Here's how the part is built. I have some questions about the finished solid (model axes, mm). A direction names the side the tool comes from. Coordinates: 2 decimals unless noted, no trailing zeros. Order: outer loops, then holes, each group sorted by start corner. A loop starts at its lowest first (then second) coordinate and runs counter-clockwise, first axis right, second up. Notation, with made-up numbers: (9, 11.5) - (40, 11.5) arc R22 ccw to (40, 40.5) - close; hole circle Ø3 at (68.5, -23.75). An arc over 180 degrees is marked (long way). Answer as CSV lines item,"result". Start each with the question number.
Item 1: I need wall thicknesses on line 1 (Z direction, x = -4, y = 2); line 2 (Z direction, x = -54, y = 4.75); line 3 (Z direction, x = -21.5, y = 6). Which ranges of each line are inside material? Lowest first, please.
Item 2: I'm going to push a flat-ended pin straight in: pin 1 (8 mm diameter, centred on x = -29.5, z = 8.5, fed in from +Y). Where does the tip first touch, or does it pass through?
Item 3: Imagine slicing it at D-D on x = -40. List the corners of the cut face in (y, z) for me, and give its area (3 significant figures).
Item 4: Imagine slicing it at C-C on y = 1. Count the separate pieces of the cut face and the enclosed holes in it, and give its area (3 significant figures).
Item 5: Imagine slicing it at A-A on x = -14. List the corners of the cut face in (y, z) for me.
Item 6: On a 3-axis mill with a long thin cutter (end or side, diameter ignored), from which of +Z, -Z, +X, -X, +Y, -Y can I reach the whole of each face in a straight line? I mean faces 1 (the face through (-31, 0, 32)), 2 (the face through (-5, 4, 19)). Say none if no direction works.
Item 7: Imagine slicing it at B-B on z = 4. List the corners of the cut face in (x, y) for me.
Item 8: We'd pull the mould along X, two halves only. Please class faces 3 (the face through (0, 4, 19)), 4 (the face through (-12.8, 4.2, 34.9)), 5 (the face through (-31, 4, 0)): pulls with the +X half, pulls with the -X half, needs draft (parallel to the pull), parting line crosses it, or undercut.
Autodesk Inventor part; units mm, degrees
ref_plane "YZ Plane" through (0, 0, 0) normal (1, 0, 0) x (0, 1, 0)
ref_plane "XZ Plane" through (0, 0, 0) normal (0, 1, 0) x (-1, 0, 0)
ref_plane "XY Plane" through (0, 0, 0) normal (0, 0, 1) x (1, 0, 0)
sketch "スケッチ1" plane through (0, 0, 0) normal (0, 1, 0) x (-1, 0, 0)
  circle A0 centre (4, 34) radius 1.5
  circle A1 centre (44, 34) radius 1.5
  circle A2 centre (24, 34) radius 1.5
  circle A3 centre (44, 4) radius 1.5
  circle A4 centre (24, 4) radius 1.5
  circle A5 centre (4, 4) radius 1.5
  circle A6 centre (14, 4) radius 1.5
  circle A7 centre (34, 4) radius 1.5
  circle A8 centre (54, 4) radius 1.5
  circle A9 centre (34, 34) radius 1.5
  circle A10 centre (54, 34) radius 1.5
  circle A11 centre (14, 34) radius 1.5
  line L0 (0, 0) -> (62, 0)
  line L1 (62, 0) -> (62, 38)
  line L2 (62, 38) -> (0, 38)
  line L3 (0, 38) -> (0, 0)
extrude "押し出し1" add sketch "スケッチ1" along normal blind 8.5
sketch "スケッチ2" plane through (0, 0, 0) normal (0, -1, 0) x (1, 0, 0)
  line L0 (0, 0) -> (-62, 0)
  line L1 (0, 38) -> (0, 0)
  line L2 (-62, 38) -> (0, 38)
  line L3 (-62, 0) -> (-62, 38)
  line L4 (-57, 30) -> (-5, 30)
  line L5 (-5, 30) -> (-5, 8)
  line L6 (-5, 8) -> (-57, 8)
  line L7 (-57, 8) -> (-57, 30)
  dimension "d2" = 5
  dimension "d3" = 5
  dimension "d4" = 8
  dimension "d5" = 8
extrude "押し出し2" cut sketch "スケッチ2" against normal through all contours L4 L5 L6 L7
properties part number "知能ロボコンタミヤギアモータ用マウントスペーサ"
Responses:
1,line 1,"z = 0 to 2.5, 5.5 to 32.5, 35.5 to 38"
1,line 2,"z = 0 to 2.5, 5.5 to 8, 30 to 32.5, 35.5 to 38"
1,line 3,"z = 0 to 8, 30 to 38"
2,pin 1,"stops at y = 8.5"
3,outline,"(0, 0) - (8.5, 0) - (8.5, 8) - (0, 8) - close; (0, 30) - (8.5, 30) - (8.5, 38) - (0, 38) - close"
3,area,"136 mm^2"
4,separate pieces,"1"
4,enclosed holes,"13"
4,area,"1,130 mm^2"
5,outline,"(0, 0) - (8.5, 0) - (8.5, 2.5) - (0, 2.5) - close; (0, 5.5) - (8.5, 5.5) - (8.5, 8) - (0, 8) - close; (0, 30) - (8.5, 30) - (8.5, 32.5) - (0, 32.5) - close; (0, 35.5) - (8.5, 35.5) - (8.5, 38) - (0, 38) - close"
6,face 1,"+Z, -Z, +X, -X, -Y"
6,face 2,"+Y, -Y"
7,outline,"(-62, 0) - (-55.5, 0) - (-55.5, 8.5) - (-62, 8.5) - close; (-52.5, 0) - (-45.5, 0) - (-45.5, 8.5) - (-52.5, 8.5) - close; (-42.5, 0) - (-35.5, 0) - (-35.5, 8.5) - (-42.5, 8.5) - close; (-32.5, 0) - (-25.5, 0) - (-25.5, 8.5) - (-32.5, 8.5) - close; (-22.5, 0) - (-15.5, 0) - (-15.5, 8.5) - (-22.5, 8.5) - close; (-12.5, 0) - (-5.5, 0) - (-5.5, 8.5) - (-12.5, 8.5) - close; (-2.5, 0) - (0, 0) - (0, 8.5) - (-2.5, 8.5) - close"
8,face 3,"pulls with the +X half"
8,face 4,"undercut"
8,face 5,"needs draft"
